Geometry check sheet. Reference: the model listing, model coordinates, mm. A direction names the side the tool comes from. Coordinates: 2 decimals unless noted, no trailing zeros. Write each loop counter-clockwise with the first axis right and the second up, starting at its lowest first coordinate (ties: lowest second). Pieces come first, ordered by that corner, then holes. Notation, with made-up numbers: (76, 55.25) -> (85, 55.25) arc R16 ccw to (85, 65.25) -> close; hole circle Ø8 at (-22.5, -27). An arc over 180 degrees is marked (long way). Answer in a Markdown table with one row per item. Add a question column.
1. Cross-section at B-B on x = 5.5. Record the cut outline in (y, z).
2. Cross-section at D-D on x = 12.25. Record the cut outline in (y, z), and give its area (3 significant figures).
3. Depth check by flat-ended pin: P1, Ø5.5, axis at y = 150.33, z = 30, coming from the +X side; P2, Ø9, axis at x = 4, y = 104.5, coming from the +Z side; P3, Ø2, axis at y = 151, z = 10, coming from the +X side; P4, Ø3, axis at x = 0.5, z = 9.5, coming from the +Y side. Enter the tip coordinate at first touch or a pass-through.
4. Mould release check, pull along Z, two halves, no side actions. Record for faces 5 (the cylindrical face through (11.16, 148.33, 9.56)), 6 (the flat face through (13, 160.33, 20)), 7 (the flat face through (14.204, 149, 28)), 8 (the flat face through (3, 10, 10)): pulls with the +Z half, pulls with the -Z half, needs draft (parallel to the pull), parting line crosses it, or undercut.
5. Set-up check for faces 1 (the flat face through (3, 40.33, 24)), 2 (the flat face through (3, -25.67, 20)), 3 (the cylindrical face through (16.23, 154.05, 30.49)), 4 (the flat face through (8.204, 150, 20)): record each of +Z, -Z, +X, -X, +Y, -Y from which the full face is reachable in a straight line by a thin tool's end or side.
6. Cross-section at A-A on z = 30. Record the cut outline in (x, y).
7. Cross-section at C-C on z = 16. Record the cut outline in (x, y).
8. Scan lines: L1, parallel to Y at x = 16, z = 30; L2, parallel to Y at x = 13.5, z = 38; L3, parallel to Z at x = 15.5, y = -14. Record each from-to range of solid material in increasing order. Write a range as from..to.
```python
from build123d import *

# Parameters (mm, degrees)
SKETCH_1_W          = 30
SKETCH_1_H          = 186
EXTRUDE_1_DEPTH     = 10
SKETCH_2_W          = 30
SKETCH_2_H          = 5
SKETCH_2_H_2        = 20
EXTRUDE_2_DEPTH     = 30
FILLET_1_R          = 2.5
FILLET_4_R          = 10
CHAMFER_7_SIZE      = 10
SKETCH_3_W          = 40
SKETCH_3_H          = 20
CUT_EXTRUDE_1_DEPTH = 20
SKETCH_7_R          = 2.05
CUT_EXTRUDE_3_DEPTH = 10
SKETCH_8_R          = 3.75
CUT_EXTRUDE_4_DEPTH = 4


with BuildPart() as part:
    # 草圖1 → 填料-伸長1 (new body)
    with BuildSketch(Plane.XY):
        with Locations((3.2037008, 67.330357143)):
            Rectangle(SKETCH_1_W, SKETCH_1_H)
    extrude(amount=EXTRUDE_1_DEPTH)

    # 草圖2 → 填料-伸長2 (add)
    with BuildSketch(Plane.XY.offset(10)):
        with Locations((3.2037008, -23.169642857)):
            Rectangle(SKETCH_2_W, SKETCH_2_H)
        with Locations((3.2037008, 42.830357143)):
            Rectangle(SKETCH_2_W, SKETCH_2_H)
        with Locations((3.2037008, 150.330357143)):
            Rectangle(SKETCH_2_W, SKETCH_2_H_2)
    extrude(amount=EXTRUDE_2_DEPTH)

    # 圓角1
    fillet_1_edges = [part.edges().sort_by_distance(p)[0] for p in [
        (3.2037008, -20.669642857, 40),
        (3.2037008, 40.330357143, 40),
    ]]
    fillet(fillet_1_edges, radius=FILLET_1_R)

    # 圓角4
    fillet_4_edges = [part.edges().sort_by_distance(p)[0] for p in [
        (3.2037008, 45.330357143, 10),
    ]]
    fillet(fillet_4_edges, radius=FILLET_4_R)

    # 導角7
    chamfer_7_edges = [part.edges().sort_by_distance(p)[0] for p in [
        (3.2037008, 140.330357143, 10),
    ]]
    chamfer(chamfer_7_edges, length=CHAMFER_7_SIZE)

    # 草圖3 → 除料-伸長1 (cut)
    with BuildSketch(Plane.ZY.offset(11.7962992)):
        with Locations((20, 150.330357143)):
            Rectangle(SKETCH_3_W, SKETCH_3_H)
    extrude(amount=-CUT_EXTRUDE_1_DEPTH, mode=Mode.SUBTRACT)

    # 草圖7 → 除料-伸長3 (cut)
    with BuildSketch(Plane.ZY.offset(-8.2037008)):
        with Locations((30, 150.330357143)):
            Circle(SKETCH_7_R)
        with Locations((10, 150.330357143)):
            Circle(SKETCH_7_R)
    extrude(amount=-CUT_EXTRUDE_3_DEPTH, mode=Mode.SUBTRACT)

    # 草圖8 → 除料-伸長4 (cut)
    with BuildSketch(Plane(origin=(18.2037008, 0, 0), x_dir=(0, 0, -1), z_dir=(1, 0, 0))):
        with Locations((-30, 150.330357143)):
            Circle(SKETCH_8_R)
        with Locations((-10, 150.330357143)):
            Circle(SKETCH_8_R)
    extrude(amount=-CUT_EXTRUDE_4_DEPTH, mode=Mode.SUBTRACT)


solid = part.part
```
Results found:
| question | item | result |
|---|---|---|
| 1 | outline | (-25.67, 0) -> (140.33, 0) -> (140.33, 20) -> (130.33, 10) -> (55.33, 10) arc R10 cw to (45.33, 20) -> (45.33, 40) -> (42.83, 40) arc R2.5 ccw to (40.33, 37.5) -> (40.33, 10) -> (-20.67, 10) -> (-20.67, 37.5) arc R2.5 ccw to (-23.17, 40) -> (-25.67, 40) -> close |
| 2 | outline | (-25.67, 0) -> (160.33, 0) -> (160.33, 40) -> (140.33, 40) -> (140.33, 20) -> (130.33, 10) -> (55.33, 10) arc R10 cw to (45.33, 20) -> (45.33, 40) -> (42.83, 40) arc R2.5 ccw to (40.33, 37.5) -> (40.33, 10) -> (-20.67, 10) -> (-20.67, 37.5) arc R2.5 ccw to (-23.17, 40) -> (-25.67, 40) -> close; hole circle Ø4.1 at (150.33, 10); hole circle Ø4.1 at (150.33, 30) |
| 2 | area | 2,800 mm^2 |
| 3 | P1 | stops at x = 14.2 |
| 3 | P2 | stops at z = 10 |
| 3 | P3 | passes through |
| 3 | P4 | stops at y = 140.33 |
| 4 | face 5 | undercut |
| 4 | face 6 | needs draft |
| 4 | face 7 | undercut |
| 4 | face 8 | pulls with the +Z half |
| 5 | face 1 | +Z, +X, -X |
| 5 | face 2 | +Z, -Z, +X, -X, -Y |
| 5 | face 3 | +X |
| 5 | face 4 | +Z, -Z, -X, +Y |
| 6 | outline | (-11.8, -25.67) -> (18.2, -25.67) -> (18.2, -20.67) -> (-11.8, -20.67) -> close; (-11.8, 40.33) -> (18.2, 40.33) -> (18.2, 45.33) -> (-11.8, 45.33) -> close; (8.2, 140.33) -> (18.2, 140.33) -> (18.2, 146.58) -> (14.2, 146.58) -> (14.2, 148.28) -> (8.2, 148.28) -> close; (8.2, 152.38) -> (14.2, 152.38) -> (14.2, 154.08) -> (18.2, 154.08) -> (18.2, 160.33) -> (8.2, 160.33) -> close |
| 7 | outline | (-11.8, -25.67) -> (18.2, -25.67) -> (18.2, -20.67) -> (-11.8, -20.67) -> close; (-11.8, 40.33) -> (18.2, 40.33) -> (18.2, 46.17) -> (-11.8, 46.17) -> close; (-11.8, 136.33) -> (18.2, 136.33) -> (18.2, 160.33) -> (8.2, 160.33) -> (8.2, 140.33) -> (-11.8, 140.33) -> close |
| 8 | L1 | y = -25.67..-20.67, 40.33..45.33, 140.33..146.58, 154.08..160.33 |
| 8 | L2 | y = -25.67..-20.72, 40.38..45.33, 140.33..160.33 |
| 8 | L3 | z = 0..10 |
